```python
from build123d import *

# Parameters (mm, degrees)
F0_R     = 3.175
F1_DEPTH = 50.8
F3_DEPTH = 3.175
F4_R     = 2.3876


with BuildPart() as f1:
    # F0 (on Front) → F1 (new body, symmetric)
    with BuildSketch(Plane.XZ):
        Circle(F0_R)
    extrude(amount=F1_DEPTH, both=True)

    # F2 (on Right) → F3 (join, symmetric)
    with BuildSketch(Plane.YZ):
        with BuildLine():
            Line((-44.45, -3.175), (-44.45, 3.175))
            Line((-44.45, 3.175), (-62.426432, 6.25859))
            ThreePointArc((-62.426432, 6.25859), (-69.85, 0), (-62.426432, -6.25859))
            Line((-62.426432, -6.25859), (-44.45, -3.175))
        make_face()
    extrude(amount=F3_DEPTH, both=True)

    # F4
    f4_edges = [f1.edges().sort_by_distance(p)[0] for p in [
        (3.175, -69.85, 0),
        (-3.175, -69.85, 0),
    ]]
    fillet(f4_edges, radius=F4_R)


solid = f1.part
```
Here's how the part is built. I have some questions about the finished solid (model axes, mm). A direction names the side the tool comes from. Round coordinates to 2 decimals unless told otherwise and drop trailing zeros. Order: outer loops, then holes, each group sorted by start corner. A loop starts at its lowest first (then second) coordinate and runs counter-clockwise, first axis right, second up. Notation, with made-up numbers: M -30.5,58.5 L 22.5,58.5 A32 ccw 22.5,94.5 Z; hole C -2,3.25 d3. An arc over 180 degrees is marked long. One line per question, with ' | ' between items.
1) For faces 1 (the face through (2.42, -44.45, -2.3)), 2 (the face through (-2.29, -44.45, -2.42)), 3 (the face through (2.3, -44.45, 2.403)), which set-ups out of +Z, -Z, +X, -X, +Y, -Y let a thin tool reach every point of the face, with its end or its side?
Working result:
face 1: -Z, +X, +Y | face 2: -Z, -X, +Y | face 3: +Z, +X, +Y
2) For pin 1 Ø1 at (x, y) = (2, -55) entering from -Z; pin 2 Ø2.5 at (x, z) = (2.5, 2.5) entering from +Y, each with a flat end and sliding along its axis, tell me the tip position at first contact or that it passes through.
Working result:
pin 1: z = -4.9 | pin 2: y = 50.8
3) I want a section at A-A, the plane y = 25.5. Write out the boundary of the cut face in (x, z) (3 decimals).
Working result:
outline: C 0,0 d6.35
4) I want a section at B-B, the plane x = 2. Write out the boundary of the cut face in (y, z), then the cut area to 3 significant figures.
Working result:
outline: M -62.48,-5.93 L -44.45,-2.84 L -44.45,-2.47 L 50.8,-2.47 L 50.8,2.47 L -44.45,2.47 L -44.45,2.84 L -62.48,5.93 A6.02 ccw long Z | area: 697 mm²
5) I need wall thicknesses on line 1 along Y through (x, z) = (1, 0.25); line 2 along X through (y, z) = (-8, -0.25). Which ranges of each line are inside material? Lowest first, please.
Working result:
line 1: -69.84 to 50.8 | line 2: -3.17 to 3.17
